```python
from build123d import *

# Parameters (mm, degrees)
F2_R         = 84.15
F3_DEPTH     = 535
F5_D         = 137.8
F3_FACE1_R   = 84.15
F3_FACE1_R_2 = 68.9


with BuildPart() as f1:
    # F0 (on Front) → F1 (revolve)
    with BuildSketch(Plane.XZ):
        with BuildLine():
            Line((86.0478096959, 0), (0, 0))
            Line((0, 0), (0, -50))
            Line((0, -50), (131.6733765197, -50))
            ThreePointArc((131.6733765197, -50), (145.185180672, -44.7455467362), (151.5972704815, -31.743114855))
            Line((151.5972704815, -31.743114855), (193.744331763, 450))
            Line((193.744331763, 450), (193.744331763, 1022.2607851028))
            Line((193.744331763, 1022.2607851028), (0, 1022.2607851028))
            Line((0, 1022.2607851028), (0, 892.1018242836))
            Line((0, 892.1018242836), (143.744331763, 892.1018242836))
            Line((143.744331763, 892.1018242836), (143.744331763, 450))
            Line((143.744331763, 450), (105.9717036578, 18.256885145))
            ThreePointArc((105.9717036578, 18.256885145), (99.5596138483, 5.2544532638), (86.0478096959, 0))
        make_face()
    revolve(axis=Axis((0, 0, -25), (0, 0, -1)))

    # F2 (on Right) → F3 (join, symmetric)
    with BuildSketch(Plane.YZ):
        with Locations((0, 200)):
            Circle(F2_R)
    extrude(amount=F3_DEPTH, both=True)

    # F5 (through all)
    with Locations(Plane(origin=(-535, 0, 0), x_dir=(0, -1, 0), z_dir=(-1, 0, 0))):
        with Locations((0, 200)):
            Hole(F5_D / 2)

    # F8: sweep along a path in F7
    with BuildLine(Plane(origin=(0, 0, 0), x_dir=(-1, 0, 0), z_dir=(0, 1, 0))) as f8_path:
        ThreePointArc((-535, 200), (-622.4814326387, 182.5988611321), (-696.6446101792, 133.0446101792))
    # F3_face1 (on face) → F8 (sweep)
    with BuildSketch(Plane(origin=(535, 0, 200), x_dir=(0, 1, 0), z_dir=(1, 0, 0))):
        Circle(F3_FACE1_R)
        Circle(F3_FACE1_R_2, mode=Mode.SUBTRACT)
    sweep(path=f8_path.line)


solid = f1.part
```
Check sheet for the modelled part. Datum: model origin and axes. Units: mm. A direction names the side the tool comes from. Coordinates: 2 decimals unless noted, no trailing zeros. Order: outer loops, then holes, each group sorted by start corner. A loop starts at its lowest first (then second) coordinate and runs counter-clockwise, first axis right, second up. Notation, with made-up numbers: M 84.5,-31.5 L 111.5,-31.5 A26 ccw 111.5,-7.5 Z; hole C 86,71.5 d2. An arc over 180 degrees is marked long. Write each question's results on one line, items separated by ' | '. Start each with the question number.
1. Cross-section at D-D on y = 42. State how many separate pieces and enclosed holes the cut face has, and give its area (3 significant figures).
2. Cross-section at C-C on z = 514. Record the cut outline in (x, y).
3. Mould release check, pull along Z, two halves, no side actions. Record for faces 4 (the face through (178.97, 74.21, 740.14)), 5 (the face through (7.49, -14.94, 132.74)), 6 (the face through (719, -61.9, 155.4)): +Z half, -Z half, draft (parallel to the pull), parting line (faces both ways), or undercut.
4. Cross-section at A-A on x = 0. Record the cut outline in (y, z), and give its area (3 significant figures).
5. Access from +Z, -Z, +X, -X, +Y, -Y to the whole of each face (thin tool, end or side, straight path). Record for faces 1 (the face through (-339.3, -18.24, 117.85)), 2 (the face through (-18.71, -142.52, 667.96)), 3 (the face through (2, -2, -50)).
6. Cross-section at B-B on x = 216. Record the cut outline in (y, z).
7. Material ranges on probe 1 along Y at (x, z) = (0, 614); probe 2 along Z at (x, y) = (-60, 0), recorded low to high.
8. Go/stop test with flat-tipped pins: P1, Ø8, axis at y = -48, z = 497, coming from the -X side; P2, Ø1.5, axis at y = -71, z = 276, coming from the +X side; P3, Ø4, axis at x = -292, y = -24.5, coming from the -Z side. Record where each tip stops, or that it passes through.
Checks:
1) separate pieces: 2 | enclosed holes: 2 | area: 187,000 mm²
2) outline: C 0,0 d387.49; hole C 0,0 d287.49
3) face 4: draft | face 5: undercut | face 6: -Z half
4) outline: M -193.74,450 L -151.6,-31.74 A20 ccw -131.67,-50 L 131.67,-50 A20 ccw 151.6,-31.74 L 193.74,450 L 193.74,1022.26 L -193.74,1022.26 Z; C 0,200 d168.3; hole M -143.74,450 L -105.97,18.26 A20 ccw -86.05,0 L 86.05,0 A20 ccw 105.97,18.26 L 143.74,450 L 143.74,892.1 L -143.74,892.1 Z; hole C 0,200 d137.8 | area: 162,000 mm²
5) face 1: -X | face 2: none | face 3: -Z, +X, -X, +Y, -Y
6) outline: C 0,200 d168.3; hole C 0,200 d137.8
7) probe 1: y = -193.74 to -143.74, 143.74 to 193.74 | probe 2: z = -50 to 0, 115.85 to 131.1, 268.9 to 284.15, 892.1 to 1022.26
8) P1: stops at x = -188.68 | P2: stops at x = 164.13 | P3: stops at z = 118.91
